Read the model definition and answer for the solid it produces. Units are mm, in the model's axes. Give positions to 0.01 mm unless a question says otherwise; leave off trailing zeros. Write each loop counter-clockwise with the first axis right and the second up, starting at its lowest first coordinate (ties: lowest second). Pieces come first, ordered by that corner, then holes. Notation, with made-up numbers: (58.25, -26.75) - (94.25, -26.75) arc R20 ccw to (94.25, 6.25) - close; hole circle Ø3 at (-7.5, 59). An arc over 180 degrees is marked (long way). Use CSV: the item, a comma, the result in double quotes. Start each with the question number.
from build123d import *

# Parameters (mm, degrees)
SKETCH1_R           = 3.175
SKETCH1_R_2         = 3.2639
SKETCH1_R_3         = 3.96875
BOSS_EXTRUDE1_DEPTH = 3.175


with BuildPart() as part:
    # Sketch1 → Boss-Extrude1 (new body)
    # profile 1 of 3: a face of its own
    with BuildSketch(Plane.ZY.offset(25.4)):
        with BuildLine():
            Line((-88.4975, 379.360683619), (-113.503995941, 354.868900976))
            ThreePointArc((-113.503995941, 354.868900976), (-115.701762144, 347.491113055), (-110.608164688, 341.71900808))
            Line((-110.608164688, 341.71900808), (-88.4975, 333.860683619))
            Line((-88.4975, 333.860683619), (-102.195874596, 351.845168269))
            ThreePointArc((-102.195874596, 351.845168269), (-103.980307482, 357.263971701), (-102.037425504, 362.628003857))
            Line((-102.037425504, 362.628003857), (-88.4975, 379.360683619))
        make_face()
        with Locations((-107.95, 349.198183619)):
            Circle(SKETCH1_R, mode=Mode.SUBTRACT)
    # profile 2 of 3: a face of its own
    with BuildSketch(Plane.ZY.offset(25.4)):
        with BuildLine():
            Line((-54.275, 333.860683619), (-54.275, 379.360683619))
            Line((-54.275, 379.360683619), (-88.4975, 379.360683619))
            Line((-88.4975, 379.360683619), (-102.037425504, 362.628003857))
            ThreePointArc((-102.037425504, 362.628003857), (-103.980307482, 357.263971701), (-102.195874596, 351.845168269))
            Line((-102.195874596, 351.845168269), (-88.4975, 333.860683619))
            Line((-88.4975, 333.860683619), (-54.275, 333.860683619))
        make_face()
        with Locations((-83.735, 340.735683619)):
            Circle(SKETCH1_R_2, mode=Mode.SUBTRACT)
        with Locations((-95.25, 357.135683619)):
            Circle(SKETCH1_R_3, mode=Mode.SUBTRACT)
        with Locations((-60.625, 366.135683619)):
            Circle(SKETCH1_R_2, mode=Mode.SUBTRACT)
        with Locations((-83.735, 372.485683619)):
            Circle(SKETCH1_R_2, mode=Mode.SUBTRACT)
        with Locations((-60.625, 347.085683619)):
            Circle(SKETCH1_R_2, mode=Mode.SUBTRACT)
    # profile 3 of 3: a face of its own
    with BuildSketch(Plane.ZY.offset(25.4)):
        with Locations((-95.25, 357.135683619)):
            Circle(SKETCH1_R_3)
    extrude(amount=BOSS_EXTRUDE1_DEPTH)


solid = part.part
(1) The part is cut by section A-A on z = -107.95. Write down the section's boundary in (x, y) (3 decimals), plus the area to 3 significant figures.
(2) Consider probe 1 along Y at (x, z) = (-25.7, -84); probe 2 along Z at (x, y) = (-27.6, 372.5) (3 decimals); probe 3 along Z at (x, y) = (-25.75, 366.5) (1 decimal). Determine where each line is inside the solid, lowest interval first.
(3) The part is cut by section D-D on x = -26.65. Give the number of separate pieces and of enclosed holes in the cut face, plus the area to 3 significant figures.
(4) The part is cut by section B-B on y = 371.5. Write down the section's boundary in (x, z) (1 decimal).
(5) Given P1, Ø1.5, axis at x = -26.5, y = 344.5, coming from the -Z side; P2, Ø1, axis at x = -28, y = 364.5, coming from the -Z side, each flat-ended and moving along its own axis, determine where each tip first touches the part or whether it passes through.
(6) The part is cut by section C-C on z = -85.5. Write down the section's boundary in (x, y) (3 decimals).
(7) For a pull along Y with two mould halves and no side action, classify faces 1 (the face through (-26.965, 347.601, -115.725)), 2 (the face through (-27, 333.861, -72)), 3 (the face through (-28.575, 357, -79)), 4 (the face through (-26.97, 346.1, -108.64)) as pulls with the +Y half, pulls with the -Y half, needs draft (parallel to the pull), parting line crosses it, or undercut.
Reported:
1,outline,"(-28.575, 340.774) - (-25.4, 340.774) - (-25.4, 346.023) - (-28.575, 346.023) - close; (-28.575, 352.373) - (-25.4, 352.373) - (-25.4, 360.309) - (-28.575, 360.309) - close"
1,area,"41.9 mm²"
2,probe 1,"333.86 to 337.48, 343.99 to 369.23, 375.74 to 379.36"
2,probe 2,"-95.502 to -86.999, -80.471 to -54.275"
2,probe 3,"-101.6 to -63.9, -57.4 to -54.3"
3,separate pieces,"1"
3,enclosed holes,"5"
3,area,"2,130 mm²"
4,outline,"(-28.6, -96.5) - (-25.4, -96.5) - (-25.4, -86.8) - (-28.6, -86.8) - close; (-28.6, -80.6) - (-25.4, -80.6) - (-25.4, -54.3) - (-28.6, -54.3) - close"
5,P1,"z = -114.84"
5,P2,"z = -104.18"
6,outline,"(-28.575, 333.861) - (-25.4, 333.861) - (-25.4, 337.99) - (-28.575, 337.99) - close; (-28.575, 343.481) - (-25.4, 343.481) - (-25.4, 369.74) - (-28.575, 369.74) - close; (-28.575, 375.231) - (-25.4, 375.231) - (-25.4, 379.361) - (-28.575, 379.361) - close"
7,face 1,"parting line crosses it"
7,face 2,"pulls with the -Y half"
7,face 3,"needs draft"
7,face 4,"undercut"
